Read the model definition and answer for the solid it produces. Units are mm, in the model's axes. Face numbers are marked on the shaded views. A direction names the side the tool comes from. Give positions to 0.01 mm unless a question says otherwise; leave off trailing zeros. Order: outer loops, then holes, each group sorted by start corner. A loop starts at its lowest first (then second) coordinate and runs counter-clockwise, first axis right, second up.
Item 1: A cutting plane is placed at C-C (y = 4.75). State how many separate pieces and enclosed holes the cut face has, plus the area to 3 significant figures.
Item 2: Given pin 1 Ø5.5 at (x, z) = (0, 23) entering from -Y; pin 2 Ø4.5 at (y, z) = (0.5, 27.5) entering from +X; pin 3 Ø5.5 at (x, z) = (0, -23) entering from +Y, each flat-ended and moving along its own axis, determine where each tip first touches the part or whether it passes through.
Item 3: A cutting plane is placed at B-B (x = 0). Write down the section's boundary in (y, z).
Item 4: A cutting plane is placed at A-A (z = -23). Write down the section's boundary in (x, y), plus the area to 4 significant figures.
Item 5: A cutting plane is placed at D-D (z = 11.5). Write down the section's boundary in (x, y), plus the area to 3 significant figures.
Item 6: Which of the six approach directions +Z, -Z, +X, -X, +Y, -Y give full straight-line access (tool end or side, diameter ignored) to the marked faces 1, 2, 3 and 4?
Item 7: Find the intervals of material crossed by line 1 along Z through (x, y) = (-15, 3.5); line 2 along X through (y, z) = (2.5, -33.5); line 3 along X through (y, z) = (5, -9), in increasing order.
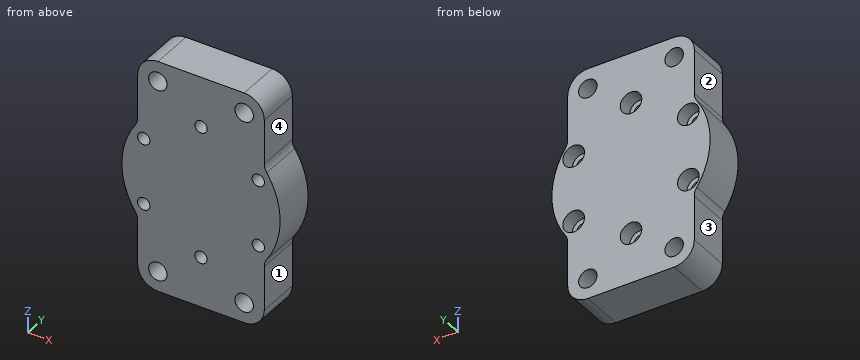
Autodesk Inventor part; units mm, degrees
ref_plane "YZ Plane" through (0, 0, 0) normal (1, 0, 0) x (0, 1, 0)
ref_plane "XZ Plane" through (0, 0, 0) normal (0, 1, 0) x (-1, 0, 0)
ref_plane "XY Plane" through (0, 0, 0) normal (0, 0, 1) x (1, 0, 0)
sketch "スケッチ1" plane through (0, 0, 0) normal (0, 1, 0) x (-1, 0, 0)
  line L0 (27.5, 27.5) -> (-27.5, 27.5)
  line L1 (-27.5, 27.5) -> (-27.5, -27.5)
  line L2 (-27.5, -27.5) -> (27.5, -27.5)
  line L3 (27.5, -27.5) -> (27.5, 27.5)
  line L4 (27.5, 27.5) -> (-27.5, -27.5) construction
  line L5 (-27.5, 27.5) -> (27.5, -27.5) construction
  line L6 (15, 33.5) -> (-15, 33.5) construction
  line L7 (-15, 33.5) -> (-15, -33.5) construction
  line L8 (-15, -33.5) -> (15, -33.5) construction
  line L9 (15, -33.5) -> (15, 33.5) construction
  line L10 (15, 33.5) -> (-15, -33.5) construction
  line L11 (-15, 33.5) -> (15, -33.5) construction
  circle A0 centre (-15, 33.5) radius 5 construction
  circle A1 centre (0, 0) radius 27.5
  line L12 (22, -40.5) -> (-22, -40.5)
  line L13 (-22, -40.5) -> (-22, 40.5)
  line L14 (-22, 40.5) -> (22, 40.5)
  line L15 (22, 40.5) -> (22, -40.5)
  line L16 (22, -40.5) -> (-22, 40.5) construction
  line L17 (-22, -40.5) -> (22, 40.5) construction
  point P0 (-22, -16.5)
  point P1 (22, -16.5)
  point P2 (22, 16.5)
  point P3 (-22, 16.5)
  dimension "d44" = 55
  dimension "d45" = 10
  dimension "d46" = 6
  dimension "d53" = 55
  dimension "d54" = 30
  dimension "d55" = 7
  dimension "d56" = 7
extrude "押し出し1" add sketch "スケッチ1" along normal mid plane 15 contours L15 A1 L0 | L0 L13 L14 L15 | A1 L15 | A1 L13 L0 | A1 L15 L13 | L15 L2 A1 | L13 A1 | L15 L12 L13 L2 | L2 L13 A1
sketch "スケッチ2" plane through (-1, 7.5, 27) normal (0, -1, 0) x (1, 0, 0)
  line L0 (-14, -60.5) -> (16, -60.5)
  line L1 (16, -60.5) -> (16, 6.5)
  line L2 (16, 6.5) -> (-14, 6.5)
  line L3 (-14, 6.5) -> (-14, -60.5)
  line L4 (-14, -60.5) -> (16, 6.5) construction
  line L5 (16, -60.5) -> (-14, 6.5) construction
  line L6 (-21, 13.5) -> (23, 13.5)
  point P0 (1, -27)
  dimension "d52" = 30
  dimension "d58" = 7
hole "穴1" at (-15, 7.5, 33.5) at (15, 7.5, 33.5) at (15, 7.5, -33.5) at (-15, 7.5, -33.5) direction (0, -1, 0) diameter 6.4 end through all
sketch "スケッチ5" plane through (-26, 7.5, 26) normal (0, 1, 0) x (1, 0, 0)
  circle A0 centre (26, 26) radius 23
  point P0 (26, 26)
  point P1 (26, 49)
  point P2 (26, 26)
  point P3 (6.0814, 37.5)
  point P4 (26, 26)
  point P5 (6.0814, 14.5)
  point P6 (26, 26)
  point P7 (26, 3)
  point P8 (26, 26)
  point P9 (45.9186, 14.5)
  point P10 (26, 26)
  point P11 (45.9186, 37.5)
  dimension "d31" = 46
  dimension "d34" = 360
hole "穴4" at (19.9186, 7.5, -11.5) at (19.9186, 7.5, 11.5) at (0, 7.5, 23) at (-19.9186, 7.5, 11.5) at (-19.9186, 7.5, -11.5) at (0, 7.5, -23) direction (0, -1, 0) diameter 4.3 end through all counterbore diameter 7.5 counterbore depth 5
fillet "フィレット2" radius 7 4 edges at (-22, 0, 40.5) (22, 0, 40.5) (22, 0, -40.5) (-22, 0, -40.5)
fillet "フィレット3" radius 5 4 edges at (-22, 0, -16.5) (-22, 0, 16.5) (22, 0, -16.5) (22, 0, 16.5)
Response values:
1. separate pieces: 1
1. enclosed holes: 10
1. area: 3,380 mm2
2. pin 1: stops at y = -7.5
2. pin 2: stops at x = 22
2. pin 3: stops at y = 2.5
3. outline: (-7.5, -40.5) - (7.5, -40.5) - (7.5, -26.75) - (2.5, -26.75) - (2.5, -25.15) - (-7.5, -25.15) - close; (-7.5, -20.85) - (2.5, -20.85) - (2.5, -19.25) - (7.5, -19.25) - (7.5, 19.25) - (2.5, 19.25) - (2.5, 20.85) - (-7.5, 20.85) - close; (-7.5, 25.15) - (2.5, 25.15) - (2.5, 26.75) - (7.5, 26.75) - (7.5, 40.5) - (-7.5, 40.5) - close
4. outline: (-22, -7.5) - (-2.15, -7.5) - (-2.15, 2.5) - (-3.75, 2.5) - (-3.75, 7.5) - (-22, 7.5) - close; (2.15, -7.5) - (22, -7.5) - (22, 7.5) - (3.75, 7.5) - (3.75, 2.5) - (2.15, 2.5) - close
4. area: 579.5 mm2
5. outline: (-24.98, -7.5) - (-22.07, -7.5) - (-22.07, 2.5) - (-23.67, 2.5) - (-23.67, 7.5) - (-24.98, 7.5) - close; (-17.77, -7.5) - (17.77, -7.5) - (17.77, 2.5) - (16.17, 2.5) - (16.17, 7.5) - (-16.17, 7.5) - (-16.17, 2.5) - (-17.77, 2.5) - close; (22.07, -7.5) - (24.98, -7.5) - (24.98, 7.5) - (23.67, 7.5) - (23.67, 2.5) - (22.07, 2.5) - close
5. area: 588 mm2
6. face 1: -Z, +X, +Y, -Y
6. face 2: +Z, -X, +Y, -Y
6. face 3: -Z, -X, +Y, -Y
6. face 4: +Z, +X, +Y, -Y
7. line 1: z = -40.5 to -36.7, -30.3 to 30.3, 36.7 to 40.5
7. line 2: x = -22 to -18.2, -11.8 to 11.8, 18.2 to 22
7. line 3: x = -25.99 to -22.71, -17.12 to 17.12, 22.71 to 25.99
